```python
from build123d import *

# Parameters (mm, degrees)
SKETCH_1_R        = 30
EXTRUDE_1_DEPTH   = 58
SKETCH_2_W        = 60
SKETCH_2_H        = 60
EXTRUDE_2_DEPTH   = 2
FILLET_1_R        = 2
SKETCH_3_W        = 77
SKETCH_3_H        = 77
EXTRUDE_3_DEPTH   = 1.5
SKETCH_4_W        = 1.5
SKETCH_4_H        = 77
EXTRUDE_4_DEPTH   = 8.5
SKETCH_5_W        = 74
SKETCH_5_H        = 1.5
EXTRUDE_5_DEPTH   = 15
SKETCH_6_R        = 3.5
EXTRUDE_6_DEPTH   = 10
SKETCH_7_R        = 8.25
EXTRUDE_7_DEPTH   = 7.7
SKETCH_8_R        = 13.65
EXTRUDE_8_DEPTH   = 7.3
HOLE_WIZARD_M41_D = 3.3


with BuildPart() as part:
    # Эскиз1 → Бобышка-Вытянуть1 (new body)
    with BuildSketch(Plane(origin=(0, 0, 0), x_dir=(1, 0, 0), z_dir=(0, 1, 0))):
        with Locations(Location((0, 0, 0), (0, 0, 90))):
            Circle(SKETCH_1_R)
    extrude(amount=EXTRUDE_1_DEPTH)

    # Эскиз2 → Бобышка-Вытянуть2 (add)
    with BuildSketch(Plane.XZ):
        Rectangle(SKETCH_2_W, SKETCH_2_H)
    extrude(amount=EXTRUDE_2_DEPTH)

    # Скругление1
    fillet_1_edges = [part.edges().sort_by_distance(p)[0] for p in [
        (30, -1, -30),
        (30, -1, 30),
        (-30, -1, 30),
        (-30, -1, -30),
    ]]
    fillet(fillet_1_edges, radius=FILLET_1_R)

    # Эскиз3 → Бобышка-Вытянуть3 (add)
    with BuildSketch(Plane.XZ.offset(2)):
        with Locations((-5.5, 2.5)):
            Rectangle(SKETCH_3_W, SKETCH_3_H)
    extrude(amount=EXTRUDE_3_DEPTH)

    # Эскиз4 → Бобышка-Вытянуть4 (add)
    with BuildSketch(Plane(origin=(0, -2, 0), x_dir=(1, 0, 0), z_dir=(0, 1, 0))):
        with Locations((32.25, -2.5)):
            Rectangle(SKETCH_4_W, SKETCH_4_H)
        with Locations((-43.25, -2.5)):
            Rectangle(SKETCH_4_W, SKETCH_4_H)
    extrude(amount=EXTRUDE_4_DEPTH)

    # Эскиз5 → Бобышка-Вытянуть5 (add)
    with BuildSketch(Plane.XZ.offset(3.5)):
        with Locations((-5.5, -35.25)):
            Rectangle(SKETCH_5_W, SKETCH_5_H)
    extrude(amount=EXTRUDE_5_DEPTH)

    # Эскиз6 → Бобышка-Вытянуть6 (add)
    with BuildSketch(Plane.XZ.offset(3.5)):
        with Locations(Location((9.5, -0.5, 0), (0, 0, 90))):
            Circle(SKETCH_6_R)
    extrude(amount=EXTRUDE_6_DEPTH)

    # Эскиз7 → Бобышка-Вытянуть7 (add)
    with BuildSketch(Plane.XZ.offset(13.5)):
        with Locations(Location((9.5, -0.5, 0), (0, 0, 90))):
            Circle(SKETCH_7_R)
    extrude(amount=EXTRUDE_7_DEPTH)

    # Эскиз8 → Бобышка-Вытянуть8 (add)
    with BuildSketch(Plane.XZ.offset(21.2)):
        with Locations(Location((9.5, -0.5, 0), (0, 0, 270))):
            Circle(SKETCH_8_R)
    extrude(amount=EXTRUDE_8_DEPTH)

    # Отверстие обработанное метчиком M41 (through all)
    with Locations(Plane(origin=(0, 0, -36), x_dir=(-1, 0, 0), z_dir=(0, 0, -1))):
        with Locations((37.5, -10.5), (-26.5, -10.5)):
            Hole(HOLE_WIZARD_M41_D / 2)


solid = part.part
```
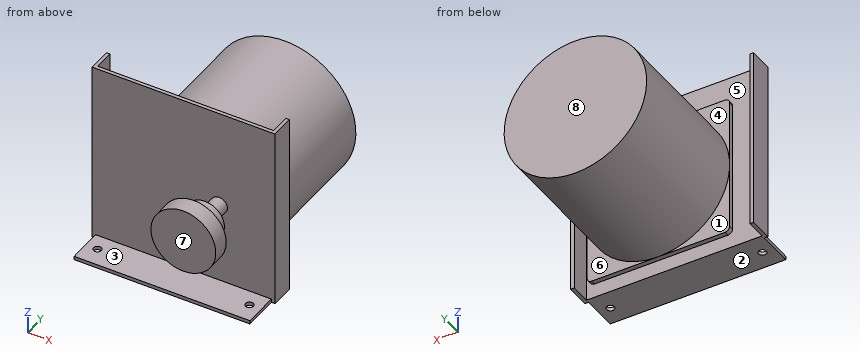
Here's how the part is built. I have some questions about the finished solid (model axes, mm). Face numbers are marked on the shaded views. A direction names the side the tool comes from. Round coordinates to 2 decimals unless told otherwise and drop trailing zeros. Write each loop counter-clockwise with the first axis right and the second up, starting at its lowest first coordinate (ties: lowest second). Pieces come first, ordered by that corner, then holes.
Q1. If we section it at C-C on z = -12: Write out the boundary of the cut face in (x, y), plus the area to 3 significant figures.
Q2. If we section it at B-B on x = -37.5: Write out the boundary of the cut face in (y, z), plus the area to 3 significant figures.
Q3. If we section it at D-D on y = 2: Write out the boundary of the cut face in (x, z), plus the area to 3 significant figures.
Q4. If we mould it in two halves opening along Z, with no side actions, what happens to the marked faces 1, 2 and 3? For each: +Z half, -Z half, draft (parallel to the pull), parting line (faces both ways), or undercut.
Q5. Will these pins go through, and if not, where does the flat tip stop? P1, Ø12, axis at x = -29.5, z = -8, coming from the +Y side; P2, Ø4, axis at x = -16.5, y = 35, coming from the -Z side; P3, Ø1.6, axis at x = -11.5, z = -35, coming from the -Y side; P4, Ø1.5, axis at y = 43.5, z = 6, coming from the +X side.
Q6. Which directions (+Z, -Z, +X, -X, +Y, -Y) give clear straight access to the entire face, cutting with the end or side of a thin tool? Please do the marked faces 4, 5, 6, 7 and 8.
Q7. If we section it at A-A on y = -10.5: Write out the boundary of the cut face in (x, z), plus the area to 3 significant figures.
Q8. Please list where these lines run through material, in increasing order: probe 1 along Y at (x, z) = (-37.5, -35.1); probe 2 along X at (y, z) = (-10, -35); probe 3 along Y at (x, z) = (-36.5, -27).
Answer below:
1. outline: (-44, -3.5) - (33, -3.5) - (33, 6.5) - (31.5, 6.5) - (31.5, -2) - (30, -2) - (30, 0) - (27.5, 0) - (27.5, 58) - (-27.5, 58) - (-27.5, 0) - (-30, 0) - (-30, -2) - (-42.5, -2) - (-42.5, 6.5) - (-44, 6.5) - close; (2.15, -28.5) - (16.85, -28.5) - (16.85, -21.2) - (2.15, -21.2) - close
1. area: 3,560 mm2
2. outline: (-18.5, -36) - (-12.15, -36) - (-12.15, -34.5) - (-18.5, -34.5) - close; (-8.85, -36) - (-2, -36) - (-2, 41) - (-3.5, 41) - (-3.5, -34.5) - (-8.85, -34.5) - close
2. area: 133 mm2
3. outline: (-44, -36) - (-42.5, -36) - (-42.5, 41) - (-44, 41) - close; circle Ø60 at (0, 0); (31.5, -36) - (33, -36) - (33, 41) - (31.5, 41) - close
3. area: 3,060 mm2
4. face 1: draft
4. face 2: -Z half
4. face 3: undercut
5. P1: stops at y = 58
5. P2: stops at z = -26.26
5. P3: stops at y = -18.5
5. P4: stops at x = 29.54
6. face 4: +Z, +Y
6. face 5: +Y
6. face 6: -Z, +Y
6. face 7: +Z, -Z, +X, -X, -Y
6. face 8: +Z, -Z, +X, -X, +Y
7. outline: (-42.5, -36) - (-39.15, -36) - (-39.15, -34.5) - (-42.5, -34.5) - close; (-35.85, -36) - (24.85, -36) - (24.85, -34.5) - (-35.85, -34.5) - close; circle Ø7 at (9.5, -0.5); (28.15, -36) - (31.5, -36) - (31.5, -34.5) - (28.15, -34.5) - close
7. area: 140 mm2
8. probe 1: y = -18.5 to -12.15, -8.85 to -2
8. probe 2: x = -42.5 to -39.07, -35.93 to 24.93, 28.07 to 31.5
8. probe 3: y = -3.5 to -2
